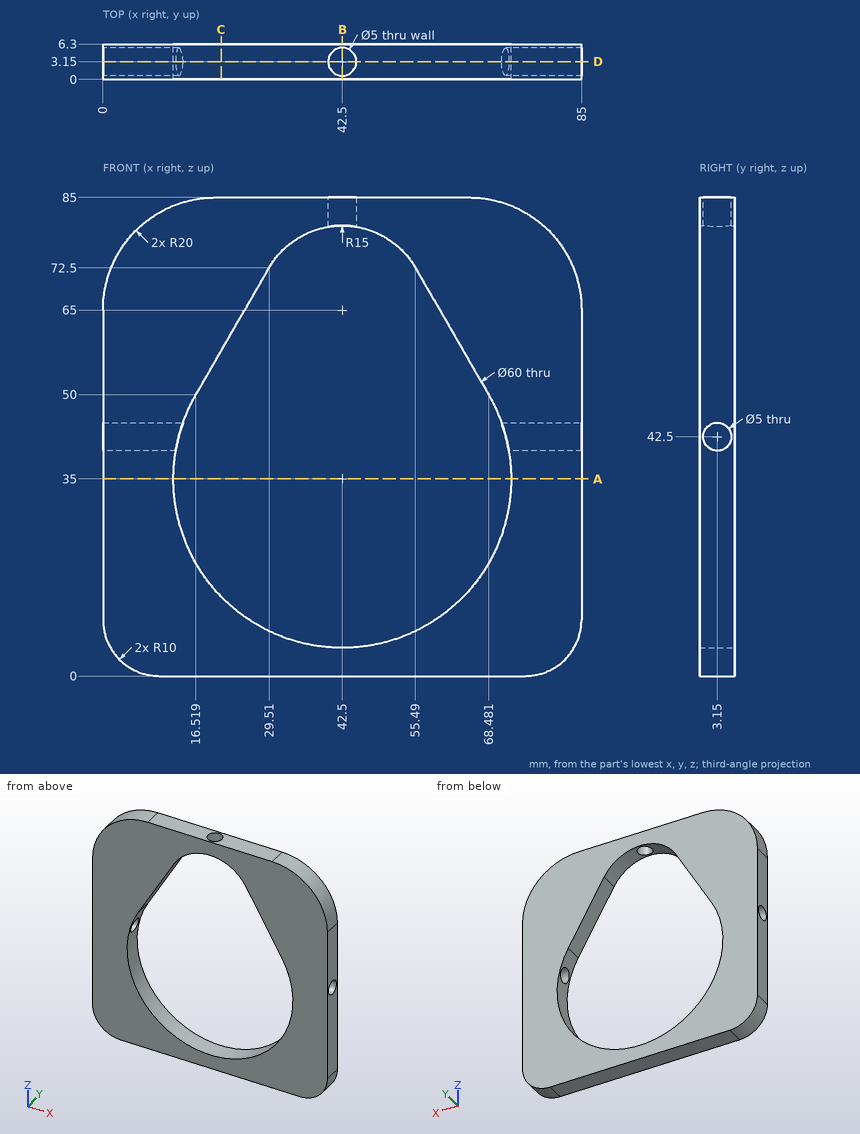
Check sheet for the drawn part. Datum: minimum x, y, z corner. Units: mm. Round coordinates to 2 decimals unless told otherwise and drop trailing zeros. Order: outer loops, then holes, each group sorted by start corner. A loop starts at its lowest first (then second) coordinate and runs counter-clockwise, first axis right, second up. Notation, with made-up numbers: M 86,38.25 L 125,38.25 A7 ccw 125,43.25 Z; hole C 12,63.25 d11. An arc over 180 degrees is marked long. Write each question's results on one line, items separated by ' | '. Start each with the question number.
1. Cross-section at A-A on z = 35. Record the boundary of the cut face in (x, y).
2. Cross-section at C-C on x = 21. Record the boundary of the cut face in (y, z), plus the area to 3 significant figures.
3. Cross-section at B-B on x = 42.5. Record the boundary of the cut face in (y, z), plus the area to 3 significant figures.
4. Cross-section at D-D on y = 3.15. Record the boundary of the cut face in (x, z) (1 decimal).
5. Material ranges on L1, parallel to Y at x = 42.5, z = 81.8; L2, parallel to X at y = 2.5, z = 36; L3, parallel to X at y = 1.25, z = 10 (1 decimal), recorded low to high. Write a range as from..to.
Resolved:
1) outline: M 0,0 L 12.5,0 L 12.5,6.3 L 0,6.3 Z; M 72.5,0 L 85,0 L 85,6.3 L 72.5,6.3 Z
2) outline: M 0,0 L 6.3,0 L 6.3,14.08 L 0,14.08 Z; M 0,57.76 L 6.3,57.76 L 6.3,85 L 0,85 Z | area: 260 mm2
3) outline: M 0,0 L 6.3,0 L 6.3,5 L 0,5 Z; M 0,80 L 0.65,80 L 0.65,85 L 0,85 Z; M 5.65,80 L 6.3,80 L 6.3,85 L 5.65,85 Z | area: 38.0 mm2
4) outline: M 0,10 A10 ccw 10,0 L 75,0 A10 ccw 85,10 L 85,40 L 72.1,40 A30 cw long 12.9,40 L 0,40 Z; M 0,45 L 14.2,45 A30 cw 16.5,50 L 29.5,72.5 A15 cw 40,79.8 L 40,85 L 20,85 A20 ccw 0,65 Z; M 45,79.8 A15 cw 55.5,72.5 L 68.5,50 A30 cw 70.8,45 L 85,45 L 85,65 A20 ccw 65,85 L 45,85 Z
5) L1: 0..0.65, 5.65..6.3 | L2: 0..12.52, 72.48..85 | L3: 0..25.9, 59.1..85
